Part print with two shaded views. Sizes in mm from the minimum x, y, z corner. Coordinates: 2 decimals unless noted, no trailing zeros. Write each loop counter-clockwise with the first axis right and the second up, starting at its lowest first coordinate (ties: lowest second). Pieces come first, ordered by that corner, then holes.
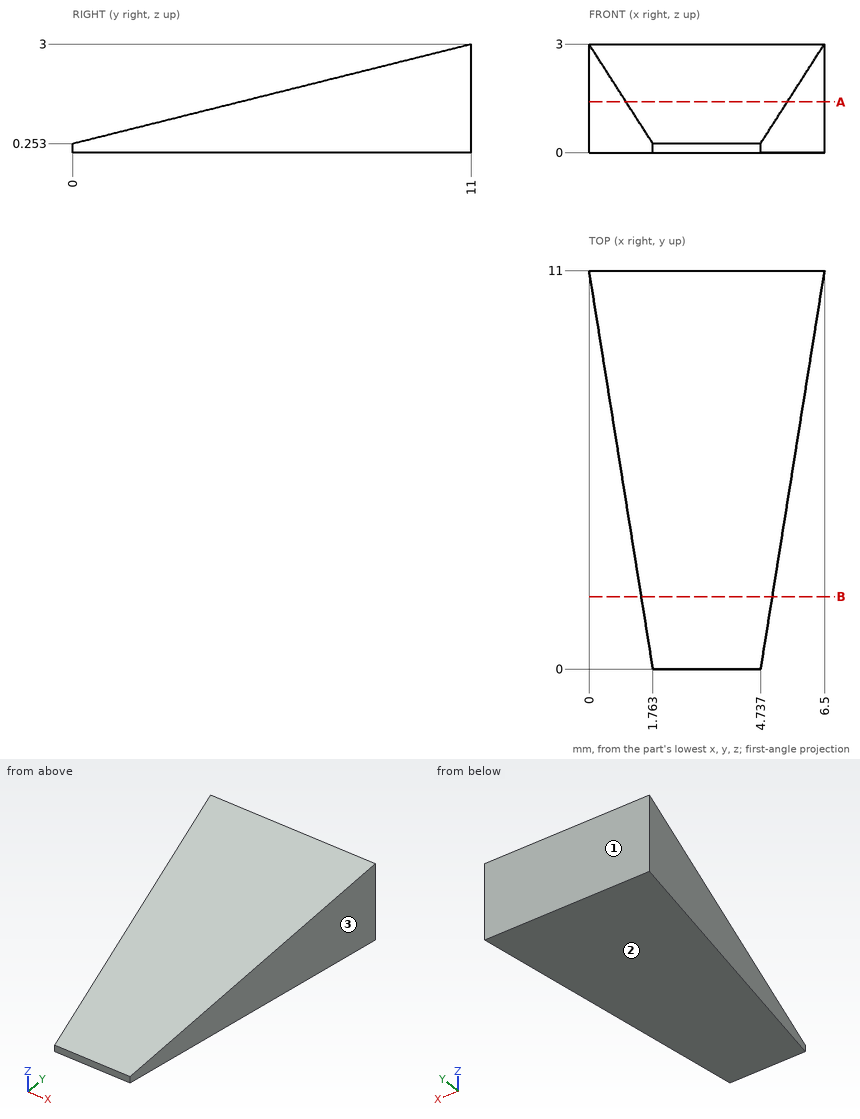
(1) Slice it at A-A, the plane z = 1.4. List the corners of the cut face in (x, y).
(2) Two-plate mould, pull along Y, no slides. Class the marked faces 1, 2 and 3: pulls with the +Y half, pulls with the -Y half, needs draft (parallel to the pull), parting line crosses it, or undercut.
(3) Probe L1, parallel to X at y = 3.75, z = 0.8; L2, parallel to Z at x = 2.5, y = 8.75; L3, parallel to X at y = 10.25, z = 0.25. List the from-to ranges inside material, lowest first.
(4) Slice it at B-B, the plane y = 2. List the corners of the cut face in (x, z).
Results:
1. outline: (0, 11) - (1.03, 4.59) - (5.47, 4.59) - (6.5, 11) - close
2. face 1: pulls with the +Y half
2. face 2: needs draft
2. face 3: pulls with the -Y half
3. L1: x = 1.16 to 5.34
3. L2: z = 0 to 2.44
3. L3: x = 0.12 to 6.38
4. outline: (1.44, 0) - (5.06, 0) - (5.06, 0.75) - (1.44, 0.75) - close
